Geometry: final body of the model. Coordinates: model frame, mm. A direction names the side the tool comes from. Round coordinates to 2 decimals unless told otherwise and drop trailing zeros. Answer as a JSON object with one key per item and string values.
from build123d import *

# Parameters (mm, degrees)
SKETCH2_R           = 3.15
BOSS_EXTRUDE1_DEPTH = 10


with BuildPart() as part:
    # Sketch2 → Boss-Extrude1 (new body)
    with BuildSketch(Plane.XY):
        Polygon((4.873707771, 0), (4.832012177, -0.636146486), (4.707640171, -1.261407971), (4.502718925, -1.865087032), (5.52904892, -2.817190886), (5.281517029, -3.257688046), (4.998967171, -3.676585913), (4.683272839, -4.071106911), (3.44623208, -3.44623208), (2.966924906, -3.866571903), (2.436853886, -4.2207551), (1.865087032, -4.502718925), (1.917572975, -5.901682854), (1.431063056, -6.038129807), (0.935064673, -6.134541988), (0.432866603, -6.190280914), (0, -4.873707771), (-0.636146486, -4.832012177), (-1.261407971, -4.707640171), (-1.865087032, -4.502718925), (-2.817190886, -5.52904892), (-3.257688046, -5.281517029), (-3.676585913, -4.998967171), (-4.071106911, -4.683272839), (-3.44623208, -3.44623208), (-3.866571903, -2.966924906), (-4.2207551, -2.436853886), (-4.502718925, -1.865087032), (-5.901682854, -1.917572975), (-6.038129807, -1.431063056), (-6.134541988, -0.935064673), (-6.190280914, -0.432866603), (-4.873707771, 0), (-4.832012177, 0.636146486), (-4.707640171, 1.261407971), (-4.502718925, 1.865087032), (-5.52904892, 2.817190886), (-5.281517029, 3.257688046), (-4.998967171, 3.676585913), (-4.683272839, 4.071106911), (-3.44623208, 3.44623208), (-2.966924906, 3.866571903), (-2.436853886, 4.2207551), (-1.865087032, 4.502718925), (-1.917572975, 5.901682854), (-1.431063056, 6.038129807), (-0.935064673, 6.134541988), (-0.432866603, 6.190280914), (0, 4.873707771), (0.636146486, 4.832012177), (1.261407971, 4.707640171), (1.865087032, 4.502718925), (2.817190886, 5.52904892), (3.257688046, 5.281517029), (3.676585913, 4.998967171), (4.071106911, 4.683272839), (3.44623208, 3.44623208), (3.866571903, 2.966924906), (4.2207551, 2.436853886), (4.502718925, 1.865087032), (5.901682854, 1.917572975), (6.038129807, 1.431063056), (6.134541988, 0.935064673), (6.190280914, 0.432866603), align=None)
        Circle(SKETCH2_R, mode=Mode.SUBTRACT)
    extrude(amount=BOSS_EXTRUDE1_DEPTH)

    # Sketch3 → Revolve1 (revolve)
    with BuildSketch(Plane(origin=(0, 0, 0), x_dir=(1, 0, 0), z_dir=(0, 1, 0))):
        Polygon((-4, 0), (-7, 0), (-7, -0.8), (-4, -2), align=None)
    revolve1 = revolve(axis=Axis((0, 0, 0), (0, 0, 1)))

    # Mirror1: Revolve1 across plane
    add(revolve1.mirror(Plane.XY.offset(5)))


solid = part.part
1) Ray query, line 1 (Y direction, x = 5.25, z = 2); line 2 (X direction, y = 2.5, z = 3); line 3 (Y direction, x = 0.25, z = 9.75). Return the intervals inside material, ascending.
Results:
{"line 1": "-3.3 to -2.56, 0.12 to 1.89", "line 2": "-5.19 to -1.92, 1.92 to 4.18", "line 3": "-7 to -3.14, 3.14 to 7"}
2) Pin query (flat end, axial travel): P1, Ø6, axis at y = -1, z = 6.5, coming from the -X side; P2, Ø3, axis at x = -5.5, z = 2, coming from the +Y side; P3, Ø5, axis at y = 1, z = 5.5, coming from the +X side. Return the tip coordinate at first contact, or that it passes through.
Results:
{"P1": "x = -7", "P2": "y = 5.28", "P3": "x = 6.19"}
3) Reachability of faces 1 (the flat face through (2.334, 5.009, 4.946)), 2 (the flat face through (1.89, -5.19, 4.95)), 3 (the flat face through (-1.89, 5.19, 4.95)), 4 (the flat face through (0.22, -5.54, 4.95)) from +Z, -Z, +X, -X, +Y, -Y: full face, straight path, thin tool, end or side. Return the list, or none.
Results:
{"face 1": "+Y", "face 2": "+X", "face 3": "-X", "face 4": "-Y"}
4) Pull-direction query (Z, two-part tool) for faces 5 (the flat face through (1.5, 3, 10)), 6 (the flat face through (5.19, 1.89, 4.95)), 7 (the flat face through (5.54, 0.22, 4.95)), 8 (the cylindrical face through (-2.5, -1.917, 4.93)); classes: +Z half, -Z half, draft (parallel to the pull), parting line (faces both ways), or undercut.
Results:
{"face 5": "+Z half", "face 6": "undercut", "face 7": "undercut", "face 8": "draft"}
